Here's how the part is built. I have some questions about the finished solid (model axes, mm). A direction names the side the tool comes from. Coordinates: 2 decimals unless noted, no trailing zeros. Write each loop counter-clockwise with the first axis right and the second up, starting at its lowest first coordinate (ties: lowest second). Pieces come first, ordered by that corner, then holes. Notation, with made-up numbers: (38.25, 39) -> (71.25, 39) arc R12 cw to (71.25, 45) -> close; hole circle Ø1 at (-6, 32.5). An arc over 180 degrees is marked (long way). Use a Markdown table: item, result. Add a question column.
```python
from build123d import *

# Parameters (mm, degrees)
ESBO_O1_R                  = 41.75
ESBO_O1_R_2                = 30.228395062
RESSALTO_EXTRUS_O1_DEPTH   = 2
ESBO_O3_R                  = 41.75
ESBO_O3_R_2                = 40.75
RESSALTO_EXTRUS_O2_DEPTH   = 1
CORTE_EXTRUS_O1_DEPTH      = 2
CORTE_EXTRUS_O1_DEPTH_BACK = 3


with BuildPart() as part:
    # Esboço1 → Ressalto-extrusão1 (new body)
    with BuildSketch(Plane(origin=(0, 0, 0), x_dir=(1, 0, 0), z_dir=(0, 1, 0))):
        Circle(ESBO_O1_R)
        Circle(ESBO_O1_R_2, mode=Mode.SUBTRACT)
    extrude(amount=RESSALTO_EXTRUS_O1_DEPTH)

    # Esboço3 → Ressalto-extrusão2 (add)
    with BuildSketch(Plane(origin=(0, 2, 0), x_dir=(1, 0, 0), z_dir=(0, 1, 0))):
        Circle(ESBO_O3_R)
        Circle(ESBO_O3_R_2, mode=Mode.SUBTRACT)
    extrude(amount=RESSALTO_EXTRUS_O2_DEPTH)

    # Esboço2 → Corte-extrusão1 (cut, two sides)
    with BuildSketch(Plane(origin=(0, 2, 0), x_dir=(1, 0, 0), z_dir=(0, 1, 0))) as corte_extrus_o1_sk:
        with BuildLine():
            Line((12.293139319, -44.064007213), (7.927300358, -28.414924055))
            ThreePointArc((7.927300358, -28.414924055), (0, -29.5), (-7.927300358, -28.414924055))
            Line((-7.927300358, -28.414924055), (-12.293139319, -44.064007213))
            ThreePointArc((-12.293139319, -44.064007213), (0, -45.746672076), (12.293139319, -44.064007213))
        make_face()
    extrude(amount=CORTE_EXTRUS_O1_DEPTH, mode=Mode.SUBTRACT)
    extrude(corte_extrus_o1_sk.sketch, amount=-CORTE_EXTRUS_O1_DEPTH_BACK, mode=Mode.SUBTRACT)


solid = part.part
```
Q1. Thinking about a two-plate mould opening in Z: for faces 4 (the flat face through (21, 0, -22)), 5 (the flat face through (-9.65, 1.19, 34.59)), 6 (the flat face through (0, 2, -31)), which applies, released by +Z, released by -Z, zero draft, split by the parting line, or undercut?
Q2. Suppose I cut it at C-C, the plane y = 1.55. Write out the boundary of the cut face in (x, z).
Q3. Suppose I cut it at A-A, the plane z = 0. Write out the boundary of the cut face in (x, y).
Q4. Please list where these lines run through material, in increasing order: line 1 (X direction, y = 2.45, z = 0); line 2 (X direction, y = 1.25, z = 0); line 3 (Y direction, x = -23.5, z = 31.5).
Q5. Suppose I cut it at B-B, the plane x = 25.5. Write out the boundary of the cut face in (y, z), and give its area (3 significant figures).
Q6. Will these pins go through, and if not, where does the flat tip stop? pin 1 (1 mm diameter, centred on x = -21.5, y = 0.5, fed in from +Z); pin 2 (1 mm diameter, centred on y = 1.5, z = 29, fed in from +X); pin 3 (1 mm diameter, centred on x = -21, z = 25, fed in from +Y).
Q7. Which directions (+Z, -Z, +X, -X, +Y, -Y) give clear straight access to the entire face, cutting with the end or side of a thin tool? Please do faces 1 (the cylindrical face through (1.677, 1.479, -41.716)), 2 (the flat face through (9.69, 1.19, 34.74)), 3 (the cylindrical face through (1.637, 2.493, -40.717)).
Q8. Suppose I cut it at D-D, the plane x = 0. Write out the boundary of the cut face in (y, z).
Answer key:
| question | item | result |
|---|---|---|
| 1 | face 4 | zero draft |
| 1 | face 5 | released by +Z |
| 1 | face 6 | undercut |
| 2 | outline | (-11.22, 40.21) arc R41.75 ccw (long way) to (11.22, 40.21) -> (8.12, 29.12) arc R30.23 cw (long way) to (-8.12, 29.12) -> close |
| 3 | outline | (-41.75, 0) -> (-30.23, 0) -> (-30.23, 2) -> (-40.75, 2) -> (-40.75, 3) -> (-41.75, 3) -> close; (30.23, 0) -> (41.75, 0) -> (41.75, 3) -> (40.75, 3) -> (40.75, 2) -> (30.23, 2) -> close |
| 4 | line 1 | x = -41.75 to -40.75, 40.75 to 41.75 |
| 4 | line 2 | x = -41.75 to -30.23, 30.23 to 41.75 |
| 4 | line 3 | y = 0 to 2 |
| 5 | outline | (0, -33.06) -> (3, -33.06) -> (3, -31.79) -> (2, -31.79) -> (2, -16.23) -> (0, -16.23) -> close; (0, 16.23) -> (2, 16.23) -> (2, 31.79) -> (3, 31.79) -> (3, 33.06) -> (0, 33.06) -> close |
| 5 | area | 69.8 mm^2 |
| 6 | pin 1 | stops at z = 36.08 |
| 6 | pin 2 | stops at x = 30.51 |
| 6 | pin 3 | stops at y = 2 |
| 7 | face 1 | +Y, -Y |
| 7 | face 2 | +Z, +Y, -Y |
| 7 | face 3 | +Y |
| 8 | outline | (0, -41.75) -> (3, -41.75) -> (3, -40.75) -> (2, -40.75) -> (2, -30.23) -> (0, -30.23) -> close |
